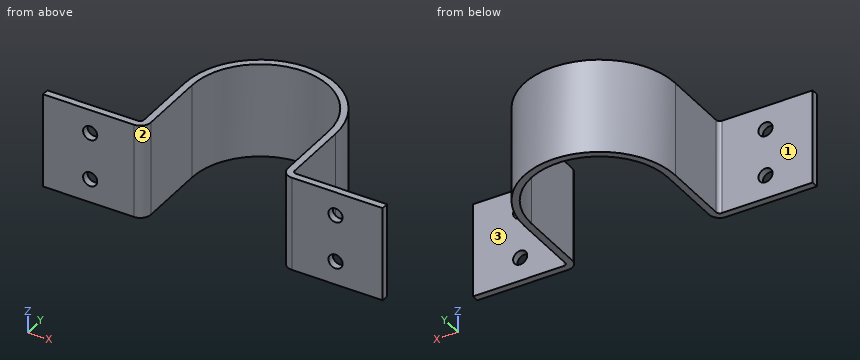
from build123d import *

# Parameters (mm, degrees)
BASE_FLANGE1_DEPTH = 20
SKETCH2_R          = 1.5
CUT_EXTRUDE1_DEPTH = 1.5
SKETCH4_R          = 1.5
CUT_EXTRUDE2_DEPTH = 1.5


# Sheet-metal steps are written as plain solids
with BuildPart() as part:
    # Sketch1 → Base-Flange1 (new body)
    with BuildSketch(Plane.XY):
        with BuildLine():
            Line((-34.427312775, 1.27753304), (-15.163912775, 1.27753304))
            ThreePointArc((-15.163912775, 1.27753304), (-14.64305792, 1.493278185), (-14.427312775, 2.01413304))
            Line((-14.427312775, 2.01413304), (-14.427312775, 16.27753304))
            ThreePointArc((-14.427312775, 16.27753304), (1.572687225, 32.27753304), (17.572687225, 16.27753304))
            Line((17.572687225, 16.27753304), (17.572687225, 2.01413304))
            ThreePointArc((17.572687225, 2.01413304), (17.78843237, 1.493278185), (18.309287225, 1.27753304))
            Line((18.309287225, 1.27753304), (37.572687225, 1.27753304))
            Line((37.572687225, 1.27753304), (37.572687225, -0.22246696))
            Line((37.572687225, -0.22246696), (18.309287225, -0.22246696))
            ThreePointArc((18.309287225, -0.22246696), (16.727772198, 0.432618013), (16.072687225, 2.01413304))
            Line((16.072687225, 2.01413304), (16.072687225, 16.27753304))
            ThreePointArc((16.072687225, 16.27753304), (1.572687225, 30.77753304), (-12.927312775, 16.27753304))
            Line((-12.927312775, 16.27753304), (-12.927312775, 2.01413304))
            ThreePointArc((-12.927312775, 2.01413304), (-13.582397749, 0.432618013), (-15.163912775, -0.22246696))
            Line((-15.163912775, -0.22246696), (-34.427312775, -0.22246696))
            Line((-34.427312775, -0.22246696), (-34.427312775, 1.27753304))
        make_face()
    extrude(amount=BASE_FLANGE1_DEPTH)

    # Sketch2 → Cut-Extrude1 (cut)
    with BuildSketch(Plane(origin=(0, 1.27753304, 0), x_dir=(1, 0, 0), z_dir=(0, 1, 0))):
        with Locations(Location((-24.427312775, -5, 0), (0, 0, 270))):
            Circle(SKETCH2_R)
        with Locations(Location((-24.427312775, -15, 0), (0, 0, 270))):
            Circle(SKETCH2_R)
    extrude(amount=-CUT_EXTRUDE1_DEPTH, mode=Mode.SUBTRACT)

    # Sketch4 → Cut-Extrude2 (cut)
    with BuildSketch(Plane(origin=(0, 1.27753304, 0), x_dir=(1, 0, 0), z_dir=(0, 1, 0))):
        with Locations(Location((27.572687225, -5, 0), (0, 0, 270))):
            Circle(SKETCH4_R)
        with Locations(Location((27.572687225, -15, 0), (0, 0, 270))):
            Circle(SKETCH4_R)
    extrude(amount=-CUT_EXTRUDE2_DEPTH, mode=Mode.SUBTRACT)


solid = part.part
The listing builds one solid part. Answer for the finished solid, in the listing's coordinates (mm). Face numbers are marked on the shaded views. A direction names the side the tool comes from. Coordinates: 2 decimals unless noted, no trailing zeros. Loops run counter-clockwise (first coordinate to the right, second up) from the corner with the lowest first, then second, coordinate; pieces in that order, holes last. Notation, with made-up numbers: M 73.5,-26.75 L 109.5,-26.75 A23 cw 109.5,-10.75 Z; hole C 84,-21.5 d5. An arc over 180 degrees is marked long. Answer in a Markdown table with one row per item.
1) Which of the six approach directions +Z, -Z, +X, -X, +Y, -Y give full straight-line access (tool end or side, diameter ignored) to the marked faces 1, 2 and 3?
Answers below:
| item | result |
|---|---|
| face 1 | +Z, -Z, -X, +Y |
| face 2 | +Z, -Z, -Y |
| face 3 | +Z, -Z, +X, +Y |
2) Find section C-C (z = 11.25). Determine the outline of the cut face in (x, y).
Answers below:
| item | result |
|---|---|
| outline | M -34.43,-0.22 L -15.16,-0.22 A2.24 ccw -12.93,2.01 L -12.93,16.28 A14.5 cw 16.07,16.28 L 16.07,2.01 A2.24 ccw 18.31,-0.22 L 37.57,-0.22 L 37.57,1.28 L 18.31,1.28 A0.74 cw 17.57,2.01 L 17.57,16.28 A16 ccw -14.43,16.28 L -14.43,2.01 A0.74 cw -15.16,1.28 L -34.43,1.28 Z |
3) Find section A-A (z = 15). Determine the outline of the cut face in (x, y), then the cut area to 3 significant figures.
Answers below:
| item | result |
|---|---|
| outline | M -34.43,-0.22 L -25.93,-0.22 L -25.93,1.28 L -34.43,1.28 Z; M -22.93,-0.22 L -15.16,-0.22 A2.24 ccw -12.93,2.01 L -12.93,16.28 A14.5 cw 16.07,16.28 L 16.07,2.01 A2.24 ccw 18.31,-0.22 L 26.07,-0.22 L 26.07,1.28 L 18.31,1.28 A0.74 cw 17.57,2.01 L 17.57,16.28 A16 ccw -14.43,16.28 L -14.43,2.01 A0.74 cw -15.16,1.28 L -22.93,1.28 Z; M 29.07,-0.22 L 37.57,-0.22 L 37.57,1.28 L 29.07,1.28 Z |
| area | 170 mm^2 |
4) Find the intervals of material crossed by probe 1 along X at (y, z) = (13.5, 5.5); probe 2 along X at (y, z) = (0.35, 15); probe 3 along X at (y, z) = (0.6, 5), in increasing order.
Answers below:
| item | result |
|---|---|
| probe 1 | -14.43 to -12.93, 16.07 to 17.57 |
| probe 2 | -34.43 to -25.93, -22.93 to -13.67, 16.81 to 26.07, 29.07 to 37.57 |
| probe 3 | -34.43 to -25.93, -22.93 to -13.43, 16.58 to 26.07, 29.07 to 37.57 |
5) Find section D-D (y = 15). Determine the outline of the cut face in (x, z), then the cut area to 3 significant figures.
Answers below:
| item | result |
|---|---|
| outline | M -14.43,0 L -12.93,0 L -12.93,20 L -14.43,20 Z; M 16.07,0 L 17.57,0 L 17.57,20 L 16.07,20 Z |
| area | 60.0 mm^2 |
6) Find section B-B (y = 22). Determine the outline of the cut face in (x, z).
Answers below:
| item | result |
|---|---|
| outline | M -13.37,0 L -11.75,0 L -11.75,20 L -13.37,20 Z; M 14.9,0 L 16.51,0 L 16.51,20 L 14.9,20 Z |
7) Given pin 1 (3 mm diameter, centred on y = 7, z = 11, fed in from +X); pin 2 (5 mm diameter, centred on y = 24.5, z = 16, fed in from -X); pin 3 (7 mm diameter, centred on y = 6, z = 5, fed in from -X), each flat-ended and moving along its own axis, determine where each tip first touches the part or whether it passes through.
Answers below:
| item | result |
|---|---|
| pin 1 | x = 17.57 |
| pin 2 | x = -13.37 |
| pin 3 | x = -14.43 |
